```python
from build123d import *

# Parameters (mm, degrees)
F1_DEPTH = 12.5
F2_R     = 1
F3_R     = 3


with BuildPart() as f1:
    # F0 (on Right) → F1 (new body, symmetric)
    with BuildSketch(Plane.YZ):
        Polygon((-28.867513, -25), (0, 25), (0, -25), (2, -25), (2, 32.464102), (-29.599564, -22.267949), (-36.135463, -18.494447), (-34.248711, -15.226497), (-35.980762, -14.226497), (-38.867513, -19.226497), align=None)
    extrude(amount=F1_DEPTH, both=True)

    # F2
    f2_edges = [f1.edges().sort_by_distance(p)[0] for p in [
        (0, 2, 32.464102),
        (0, -38.867513, -19.226497),
        (0, -28.867513, -25),
    ]]
    fillet(f2_edges, radius=F2_R)

    # F3
    f3_edges = [f1.edges().sort_by_distance(p)[0] for p in [
        (12.5, 1, -25),
        (-12.5, 1, -25),
        (12.5, -35.114737, -14.726497),
        (-12.5, -35.114737, -14.726497),
    ]]
    fillet(f3_edges, radius=F3_R)


solid = f1.part
```
Read the model definition and answer for the solid it produces. Units are mm, in the model's axes. A direction names the side the tool comes from. Round coordinates to 2 decimals unless told otherwise and drop trailing zeros. Write each loop counter-clockwise with the first axis right and the second up, starting at its lowest first coordinate (ties: lowest second). Pieces come first, ordered by that corner, then holes. Notation, with made-up numbers: (-5, 78) - (37, 78) arc R24 ccw to (37, 109) - close; hole circle Ø5 at (60, -19.5). An arc over 180 degrees is marked (long way). Use CSV: the item, a comma, the result in double quotes.
Q1. A tool of negligible diameter and unlimited length cuts with its end or side. For faces 4 (the cylindrical face through (-11.64, 1.01, -24.1)), 5 (the cylindrical face through (-11.645, -35.578, -15.501)), 6 (the flat face through (0, 0, 0)), from which of +Z, -Z, +X, -X, +Y, -Y can it reach the whole face along a straight path? Write none if from no direction.
Values:
face 4,"-Z, -X, +Y"
face 5,"+Z, -X"
face 6,"-Z, +X, -X"
Q2. Find section D-D, the plane y = -31.5. Write down the section's boundary in (x, z), then the cut area to 3 significant figures.
Values:
outline,"(-12.5, -23.48) - (12.5, -23.48) - (12.5, -21.17) - (-12.5, -21.17) - close"
area,"57.7 mm²"
Q3. Find section C-C, the plane y = -8. Write down the section's boundary in (x, z), then the cut area to 3 significant figures.
Values:
outline,"(-12.5, 11.14) - (12.5, 11.14) - (12.5, 15.14) - (-12.5, 15.14) - close"
area,"100 mm²"
Q4. Find section A-A, the plane x = -2.5. Write down the section's boundary in (y, z).
Values:
outline,"(-38.37, -18.36) arc R1 ccw to (-38, -19.73) - (-29.73, -24.5) arc R1 ccw to (-28.37, -24.13) - (0, 25) - (0, -25) - (2, -25) - (2, 28.73) arc R1 ccw to (0.13, 29.23) - (-29.6, -22.27) - (-36.14, -18.49) - (-34.25, -15.23) - (-35.98, -14.23) - close"
Q5. Straight lines are drawn through the part: line 1 along Y through (x, z) = (10.75, -19); line 2 along Y through (x, z) = (10, -17); line 3 along Y through (x, z) = (-4.5, 7). For each, find the intervals that lie inside material, in ascending order.
Values:
line 1,"y = -38.49 to -35.26, -27.71 to -25.4, 0 to 2"
line 2,"y = -37.58 to -35.27, -26.56 to -24.25, 0 to 2"
line 3,"y = -12.7 to -10.39, 0 to 2"
Q6. Find section B-B, the plane z = 12. Write down the section's boundary in (x, y), then the cut area to 3 significant figures.
Values:
outline,"(-12.5, -9.81) - (12.5, -9.81) - (12.5, -7.51) - (-12.5, -7.51) - close; (-12.5, 0) - (12.5, 0) - (12.5, 2) - (-12.5, 2) - close"
area,"108 mm²"
Q7. Determine the mould class of faces 1 (the flat face through (0, 1, -25)), 2 (the cylindrical face through (0.175, 1.241, 29.703)), 3 (the flat face through (0.18, -32.82, -20.41)) for opening direction Y: +Y half, -Y half, draft (parallel to the pull), parting line (faces both ways), or undercut.
Values:
face 1,"draft"
face 2,"parting line"
face 3,"undercut"
Q8. Each of these flat-tipped pins is pushed along its axis until it touches: pin 1 Ø12 at (x, y) = (-8, -18) entering from +Z; pin 2 Ø8 at (x, y) = (3.5, -11.5) entering from +Z; pin 3 Ø3 at (x, y) = (-3.5, -29.5) entering from -Z. Where does it stop, or does it pass through?
Values:
pin 1,"stops at z = 8.22"
pin 2,"stops at z = 16.01"
pin 3,"stops at z = -24.63"
